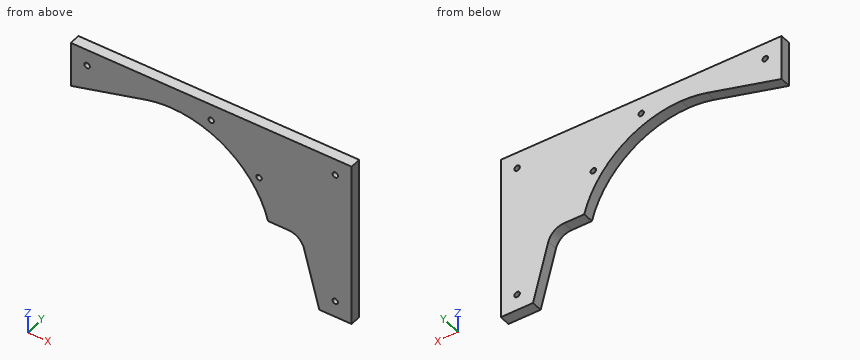
```python
from build123d import *

# Parameters (mm, degrees)
SKETCH1_R           = 3.175
BOSS_EXTRUDE1_DEPTH = 12.7
FILLET1_R           = 19.05


with BuildPart() as part:
    # Sketch1 → Boss-Extrude1 (new body)
    with BuildSketch(Plane(origin=(0, 0, 0), x_dir=(1, 0, 0), z_dir=(0, 1, 0))):
        with BuildLine():
            ThreePointArc((0, 0), (71.127685365, 24.14459572), (112.858773544, 86.59958277))
            Line((112.858773544, 86.59958277), (150.958773544, 86.59958277))
            Line((150.958773544, 86.59958277), (172.673487895, 167.64))
            Line((172.673487895, 167.64), (210.27435392, 167.64))
            Line((210.27435392, 167.64), (210.27435392, -25.4))
            Line((210.27435392, -25.4), (0, -25.4))
            Line((0, -25.4), (-117.38564608, -25.4))
            Line((-117.38564608, -25.4), (-117.38564608, 27.331720151))
            Line((-117.38564608, 27.331720151), (-30.24041723, 3.981226456))
            ThreePointArc((-30.24041723, 3.981226456), (-15.250680299, 0.999582397), (0, 0))
        make_face()
        with Locations(Location((191.22435392, -6.35, 0), (0, 0, 270))):
            Circle(SKETCH1_R, mode=Mode.SUBTRACT)
        with Locations(Location((191.22435392, 148.59, 0), (0, 0, 270))):
            Circle(SKETCH1_R, mode=Mode.SUBTRACT)
        with Locations(Location((102.32435392, 38.1, 0), (0, 0, 270))):
            Circle(SKETCH1_R, mode=Mode.SUBTRACT)
        with Locations(Location((46.44435392, -6.35, 0), (0, 0, 270))):
            Circle(SKETCH1_R, mode=Mode.SUBTRACT)
        with Locations(Location((-98.33564608, -6.35, 0), (0, 0, 270))):
            Circle(SKETCH1_R, mode=Mode.SUBTRACT)
    extrude(amount=BOSS_EXTRUDE1_DEPTH)

    # Fillet1
    fillet1_edges = [part.edges().sort_by_distance(p)[0] for p in [
        (150.958773544, 6.35, -86.59958277),
    ]]
    fillet(fillet1_edges, radius=FILLET1_R)


solid = part.part
```
The model under review builds one solid part; all positions refer to its coordinate system, in mm. Give positions to 0.01 mm unless a question says otherwise; leave off trailing zeros. Write each loop counter-clockwise with the first axis right and the second up, starting at its lowest first coordinate (ties: lowest second). Pieces come first, ordered by that corner, then holes.
(1) Consider section B-B, the plane z = -148.59. Give the boundary of the cut face in (x, y).
(2) To check wall thickness, follow L1, parallel to X at y = 5.5, z = 6.35; L2, parallel to X at y = 10.25, z = -38.1; L3, parallel to Z at x = 142, y = 9.5. State the ranges of each line that lie inside material, in increasing order.
(3) Consider section C-C, the plane y = 10.75. Give the boundary of the cut face in (x, z) (3 decimals).
(4) Consider section D-D, the plane x = 129. Give the boundary of the cut face in (y, z).
(5) Consider section A-A, the plane z = 6.35. Give the boundary of the cut face in (x, y), and give its area (3 significant figures).
(6) For P1, Ø2, axis at y = 2.5, z = -134.5, coming from the -X side; P2, Ø4, axis at y = 8.5, z = -84.5, coming from the -X side; P3, Ø4, axis at x = 122.5, y = 7, coming from the -Z side, all flat-tipped, find the tip position at first contact; note any pin that passes through.
Returned:
1. outline: (167.57, 0) - (188.05, 0) - (188.05, 12.7) - (167.57, 12.7) - close; (194.4, 0) - (210.27, 0) - (210.27, 12.7) - (194.4, 12.7) - close
2. L1: x = -117.39 to -101.51, -95.16 to 43.27, 49.62 to 188.05, 194.4 to 210.27
2. L2: x = 86.32 to 99.15, 105.5 to 210.27
2. L3: z = -87.46 to 25.4
3. outline: (-117.386, -27.332) - (-30.24, -3.981) arc R116.84 cw to (112.859, -86.6) - (136.341, -86.6) arc R19.05 cw to (154.742, -100.719) - (172.673, -167.64) - (210.274, -167.64) - (210.274, 25.4) - (-117.386, 25.4) - close; hole circle Ø6.35 at (-98.336, 6.35); hole circle Ø6.35 at (46.444, 6.35); hole circle Ø6.35 at (102.324, -38.1); hole circle Ø6.35 at (191.224, -148.59); hole circle Ø6.35 at (191.224, 6.35)
4. outline: (0, -86.6) - (12.7, -86.6) - (12.7, 25.4) - (0, 25.4) - close
5. outline: (-117.39, 0) - (-101.51, 0) - (-101.51, 12.7) - (-117.39, 12.7) - close; (-95.16, 0) - (43.27, 0) - (43.27, 12.7) - (-95.16, 12.7) - close; (49.62, 0) - (188.05, 0) - (188.05, 12.7) - (49.62, 12.7) - close; (194.4, 0) - (210.27, 0) - (210.27, 12.7) - (194.4, 12.7) - close
5. area: 3,920 mm2
6. P1: stops at x = 163.53
6. P2: stops at x = 111.68
6. P3: stops at z = -86.6
